Here's how the part is built. I have some questions about the finished solid (model axes, mm). A direction names the side the tool comes from. Round coordinates to 2 decimals unless told otherwise and drop trailing zeros. Write each loop counter-clockwise with the first axis right and the second up, starting at its lowest first coordinate (ties: lowest second). Pieces come first, ordered by that corner, then holes. Notation, with made-up numbers: (25, -18) - (62, -18) arc R8 cw to (62, -6) - close; hole circle Ø1 at (53.25, 27). An arc over 180 degrees is marked (long way). One line per question, with ' | ' between items. Start each with the question number.
(1) Imagine slicing it at A-A (z = -57). Write out the boundary of the cut face in (x, y), plus the area to 3 significant figures.
(2) If I drill on L1, parallel to Z at x = 188, y = -12; L2, parallel to Z at x = -68.5, y = -69.5; L3, parallel to Z at x = -59, y = -40, over which ranges is the centre line in solid material (lowest first)?
(3) For faces 4 (the flat face through (29, -70, 129)), 5 (the flat face through (82, 0, 41)), 6 (the flat face through (64.123, -60, 110)), which set-ups out of +Z, -Z, +X, -X, +Y, -Y let a thin tool reach every point of the face, with its end or its side?
(4) Thinking about a two-plate mould opening in X: for faces 1 (the flat face through (29, -65, 74.955)), 2 (the cylindrical face through (-91.3, -49.3, 8.4)), 3 (the cylindrical face through (189.735, -49.3, -160.586)), which applies, pulls with the +X half, pulls with the -X half, needs draft (parallel to the pull), parting line crosses it, or undercut?
(5) Imagine slicing it at B-B (y = -81). Write out the boundary of the cut face in (x, z), plus the area to 3 significant figures.
(6) Will these pins go through, and if not, where does the flat tip stop? pin 1 (3 mm diameter, centred on x = 12.5, y = -65, fed in from +Z); pin 2 (2 mm diameter, centred on y = -19, z = -8.5, fed in from -X); pin 3 (1 mm diameter, centred on y = -84.5, z = 44, fed in from +X).
from build123d import *

# Parameters (mm, degrees)
F1_DEPTH = 100
F4_DEPTH = 145
F5_W     = 129.036147
F5_H     = 6.641566
F6_DEPTH = 40
F2_R     = 75
F7_DEPTH = 319


with BuildPart() as f1:
    # F0 (on Front) → F1 (new body)
    with BuildSketch(Plane.XZ):
        with BuildLine():
            Line((175, 175), (-75, 175))
            ThreePointArc((-75, 175), (-94.36561, 155.63439), (-75, 136.26878))
            ThreePointArc((-75, 136.26878), (-62.333828, 118.8742), (-75, 101.47962))
            ThreePointArc((-75, 101.47962), (-87.223096, 87.129094), (-75, 72.778568))
            ThreePointArc((-75, 72.778568), (-60.874781, 51.035345), (-75, 29.292122))
            ThreePointArc((-75, 29.292122), (-91.304273, 7.983763), (-75, -13.324595))
            ThreePointArc((-75, -13.324595), (-54.561081, -38.546733), (-75, -63.768871))
            ThreePointArc((-75, -63.768871), (-97.317144, -82.468044), (-75, -101.167217))
            ThreePointArc((-75, -101.167217), (-54.975452, -123.345301), (-75, -145.523384))
            ThreePointArc((-75, -145.523384), (-89.738308, -160.261692), (-75, -175))
            Line((-75, -175), (175, -175))
            ThreePointArc((175, -175), (189.738308, -160.261692), (175, -145.523384))
            ThreePointArc((175, -145.523384), (157.45425, -123.345301), (175, -101.167217))
            ThreePointArc((175, -101.167217), (200.133524, -82.468044), (175, -63.768871))
            ThreePointArc((175, -63.768871), (154.578948, -31.884436), (175, 0))
            ThreePointArc((175, 0), (189.86524, 14.646061), (175, 29.292122))
            ThreePointArc((175, 29.292122), (152.58439, 51.035345), (175, 72.778568))
            ThreePointArc((175, 72.778568), (191.151996, 87.129094), (175, 101.47962))
            ThreePointArc((175, 101.47962), (156.968432, 118.8742), (175, 136.26878))
            ThreePointArc((175, 136.26878), (194.36561, 155.63439), (175, 175))
        make_face()
    extrude(amount=F1_DEPTH)

    # F3 (on face) → F4 (cut)
    with BuildSketch(Plane.XY.offset(175)):
        with BuildLine():
            Line((59.123203, -50), (-0.876797, -50))
            ThreePointArc((-0.876797, -50), (-4.412331, -51.464466), (-5.876797, -55))
            Line((-5.876797, -55), (-5.876797, -65))
            ThreePointArc((-5.876797, -65), (-4.412331, -68.535534), (-0.876797, -70))
            Line((-0.876797, -70), (59.123203, -70))
            ThreePointArc((59.123203, -70), (62.658737, -68.535534), (64.123203, -65))
            Line((64.123203, -65), (64.123203, -55))
            ThreePointArc((64.123203, -55), (62.658737, -51.464466), (59.123203, -50))
        make_face()
    extrude(amount=-F4_DEPTH, mode=Mode.SUBTRACT)

    # F5 (on face) → F6 (join)
    with BuildSketch(Plane.XZ.offset(100)):
        with Locations((5.100577, 78.275606)):
            Rectangle(F5_W, F5_H)
    extrude(amount=-F6_DEPTH)

    # F2 (on face) → F7 (cut)
    with BuildSketch(Plane.XZ.offset(100)):
        with Locations((33.149149, -25.5008)):
            Circle(F2_R)
    extrude(amount=-F7_DEPTH, mode=Mode.SUBTRACT)


solid = f1.part
Check sheet entries:
1) outline: (-62.34, -100) - (-34.92, -100) - (-34.92, 0) - (-62.34, 0) - close; (101.21, -100) - (165.16, -100) - (165.16, 0) - (101.21, 0) - close | area: 9,140 mm^2
2) L1: -167.21 to -153.32, -100.54 to -64.4, 7.49 to 21.8, 78.12 to 96.14, 141.28 to 169.99 | L2: -175 to -143.84, -102.85 to -61.45, -15.65 to 33.58, 68.49 to 105.19, 132.56 to 175 | L3: -175 to -136.12, -110.57 to -53.01, -24.08 to 175
3) face 4: +Z | face 5: +Z, -Z, +X, -X, +Y | face 6: none
4) face 1: undercut | face 2: pulls with the -X half | face 3: pulls with the +X half
5) outline: (-75, -175) - (175, -175) arc R14.74 ccw to (175, -145.52) arc R22.79 cw to (175, -101.17) arc R19.52 ccw (long way) to (175, -63.77) arc R35.1 cw to (175, 0) arc R14.65 ccw (long way) to (175, 29.29) arc R21.75 cw (long way) to (175, 72.78) arc R14.45 ccw (long way) to (175, 101.48) arc R17.41 cw (long way) to (175, 136.27) arc R19.37 ccw to (175, 175) - (-75, 175) arc R19.37 ccw to (-75, 136.27) arc R18.28 cw to (-75, 101.48) arc R14.54 ccw to (-75, 72.78) arc R23.8 cw to (-75, 29.29) arc R22.08 ccw to (-75, -13.32) arc R25.78 cw to (-75, -63.77) arc R18.99 ccw (long way) to (-75, -101.17) arc R22.29 cw to (-75, -145.52) arc R14.74 ccw to start; hole circle Ø150 at (33.15, -25.5) | area: 69,700 mm^2
6) pin 1: z = 81.6 | pin 2: x = -84.96 | pin 3: x = 153.93
